```python
from build123d import *

# Parameters (mm, degrees)
F0_R     = 11.531168
F1_DEPTH = 127
F3_D     = 8.89
F4_R     = 5.08
F5_R     = 5.08


with BuildPart() as f1:
    # F0 (on Top) → F1 (new body)
    with BuildSketch(Plane.XY):
        with Locations((-11.531168, 0)):
            Circle(F0_R)
    extrude(amount=F1_DEPTH)

    # F3 (through all)
    with Locations(Plane(origin=(0, 0, 0), x_dir=(1, 0, 0), z_dir=(0, 0, -1))):
        with Locations((-11.531168, 0)):
            Hole(F3_D / 2)

    # F4
    f4_edges = [f1.edges().sort_by_distance(p)[0] for p in [
        (-23.062335, 0, 127),
    ]]
    fillet(f4_edges, radius=F4_R)

    # F5
    f5_edges = [f1.edges().sort_by_distance(p)[0] for p in [
        (-23.062335, 0, 0),
    ]]
    fillet(f5_edges, radius=F5_R)


solid = f1.part
```
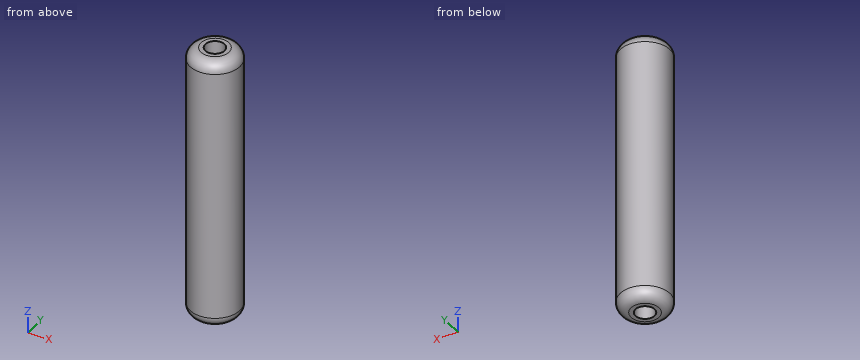
Read the model definition and answer for the solid it produces. Units are mm, in the model's axes. Coordinates: 2 decimals unless noted, no trailing zeros. Order: outer loops, then holes, each group sorted by start corner. A loop starts at its lowest first (then second) coordinate and runs counter-clockwise, first axis right, second up. Notation, with made-up numbers: (58, 41.5) - (104, 41.5) arc R16 ccw to (104, 49.5) - close; hole circle Ø8 at (41, 45.25). An arc over 180 degrees is marked (long way). Answer as a JSON object with one key per item and string values. Group by question number.
Item 1: Consider probe 1 along Y at (x, z) = (-12, 56); probe 2 along Y at (x, z) = (-7.75, 8.5); probe 3 along X at (y, z) = (-3.5, 113.5). Determine where each line is inside the solid, lowest interval first. Write a range as from..to.
Item 2: Section B-B (z = 92) is taken. Give the vertices of the cut face in (x, y) (3 decimals).
Item 3: Flat-ended cylindrical pins translate along their axes: P1, Ø5, axis at y = 5.5, z = 18, coming from the -X side; P2, Ø4, axis at x = -17, z = 68.5, coming from the -Y side; P3, Ø6, axis at y = -5, z = 90, coming from the -X side; P4, Ø7, axis at x = -11.53, y = 0, coming from the +Z side. Find the tip coordinate at first contact, or state that the pin passes through.
Item 4: Section A-A (y = 0) is taken. Give the vertices of the cut face in (x, z).
Results are:
{
 "1": {"probe 1": "y = -11.52..-4.42, 4.42..11.52", "probe 2": "y = -10.89..-2.34, 2.34..10.89", "probe 3": "x = -22.52..-14.27, -8.79..-0.54"},
 "2": {"outline": "circle Ø23.062 at (-11.531, 0); hole circle Ø8.89 at (-11.531, 0)"},
 "3": {"P1": "stops at x = -22.67", "P2": "stops at y = -11", "P3": "stops at x = -22.89", "P4": "passes through"},
 "4": {"outline": "(-23.06, 5.08) arc R5.08 ccw to (-17.98, 0) - (-15.98, 0) - (-15.98, 127) - (-17.98, 127) arc R5.08 ccw to (-23.06, 121.92) - close; (-7.09, 0) - (-5.08, 0) arc R5.08 ccw to (0, 5.08) - (0, 121.92) arc R5.08 ccw to (-5.08, 127) - (-7.09, 127) - close"}
}
